Input: part model. Units: mm. Frame: model coordinates. Round coordinates to 2 decimals unless told otherwise and drop trailing zeros. Order: outer loops, then holes, each group sorted by start corner. A loop starts at its lowest first (then second) coordinate and runs counter-clockwise, first axis right, second up.
Item 1: Line query: L1, parallel to Z at x = -63.5, y = 4.5; L2, parallel to X at y = 8.75, z = 28.5; L3, parallel to X at y = 4.5, z = 7. Output: solid intervals per line, ascending.
Item 2: Cut plane A-A on z = 1. Output: boundary loops of the cut face in (x, y).
Item 3: Cut plane B-B on y = 6. Output: boundary loops of the cut face in (x, z), then the cut area to 3 significant figures.
Item 4: Cut plane C-C on z = -121. Output: boundary loops of the cut face in (x, y).
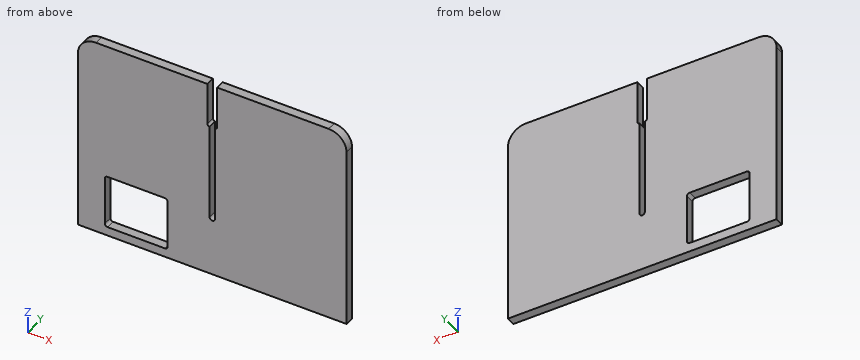
```python
from build123d import *

# Parameters (mm, degrees)
LINEAR_AUSTRAGEN1_DEPTH         = 10
VERRUNDUNG1_R                   = 20
VERRUNDUNG1_OF_SPIEGELN2_R      = 20
SKIZZE3_W                       = 70
SKIZZE3_H                       = 60
SCHNITT_LINEAR_AUSTRAGEN1_DEPTH = 11
VERRUNDUNG2_R                   = 3
SCHNITT_LINEAR_AUSTRAGEN2_DEPTH = 10


with BuildPart() as part:
    # Skizze1 → Linear austragen1 (new body)
    with BuildSketch(Plane(origin=(0, 0, 0), x_dir=(1, 0, 0), z_dir=(0, 1, 0))):
        Polygon((150, 75), (150, 150), (0, 150), (0, 75), (0, -75), (150, -75), align=None)
    linear_austragen1 = extrude(amount=LINEAR_AUSTRAGEN1_DEPTH)

    # Verrundung1
    verrundung1_edges = [part.edges().sort_by_distance(p)[0] for p in [
        (150, 5, 75),
    ]]
    fillet(verrundung1_edges, radius=VERRUNDUNG1_R)

    # Spiegeln2: Linear austragen1 across plane
    add(linear_austragen1.mirror(Plane(origin=(0, 10, -150), x_dir=(0, 0, 1), z_dir=(1, 0, 0))))

    # Verrundung1 of Spiegeln2
    verrundung1_of_spiegeln2_edges = [part.edges().sort_by_distance(p)[0] for p in [
        (-150, 5, 75),
    ]]
    fillet(verrundung1_of_spiegeln2_edges, radius=VERRUNDUNG1_OF_SPIEGELN2_R)

    # Skizze3 → Schnitt-Linear austragen1 (cut, through all)
    with BuildSketch(Plane(origin=(0, 0, 0), x_dir=(-1, 0, 0), z_dir=(0, 1, 0))):
        with Locations((85, -110)):
            Rectangle(SKIZZE3_W, SKIZZE3_H)
    extrude(amount=SCHNITT_LINEAR_AUSTRAGEN1_DEPTH, mode=Mode.SUBTRACT)

    # Verrundung2
    verrundung2_edges = [part.edges().sort_by_distance(p)[0] for p in [
        (-120, 5, -140),
        (-120, 5, -80),
        (-50, 5, -80),
        (-50, 5, -140),
    ]]
    fillet(verrundung2_edges, radius=VERRUNDUNG2_R)

    # Skizze4 → Schnitt-Linear austragen2 (cut)
    with BuildSketch(Plane.XZ):
        with BuildLine():
            Line((-3, 25), (-3, -83))
            ThreePointArc((-3, -83), (0, -86), (3, -83))
            Line((3, -83), (3, 25))
            ThreePointArc((3, 25), (4.75069059, 25.725159786), (5.475850376, 27.475850376))
            Line((5.475850376, 27.475850376), (5.475850376, 75))
            Line((5.475850376, 75), (-5.524149624, 75))
            Line((-5.524149624, 75), (-5.524149624, 27.524149624))
            ThreePointArc((-5.524149624, 27.524149624), (-4.784843316, 25.739306308), (-3, 25))
        make_face()
    extrude(amount=-SCHNITT_LINEAR_AUSTRAGEN2_DEPTH, mode=Mode.SUBTRACT)


solid = part.part
```
From the geometry:
1. L1: z = -150 to -140, -80 to 75
1. L2: x = -150 to -5.52, 5.48 to 150
1. L3: x = -150 to -3, 3 to 150
2. outline: (-150, 0) - (-3, 0) - (-3, 10) - (-150, 10) - close; (3, 0) - (150, 0) - (150, 10) - (3, 10) - close
3. outline: (-150, -150) - (150, -150) - (150, 55) arc R20 ccw to (130, 75) - (5.48, 75) - (5.48, 27.48) arc R2.48 cw to (3, 25) - (3, -83) arc R3 cw to (-3, -83) - (-3, 25) arc R2.52 cw to (-5.52, 27.52) - (-5.52, 75) - (-130, 75) arc R20 ccw to (-150, 55) - close; hole (-120, -137) arc R3 ccw to (-117, -140) - (-53, -140) arc R3 ccw to (-50, -137) - (-50, -83) arc R3 ccw to (-53, -80) - (-117, -80) arc R3 ccw to (-120, -83) - close
3. area: 61,900 mm2
4. outline: (-150, 0) - (-120, 0) - (-120, 10) - (-150, 10) - close; (-50, 0) - (150, 0) - (150, 10) - (-50, 10) - close
